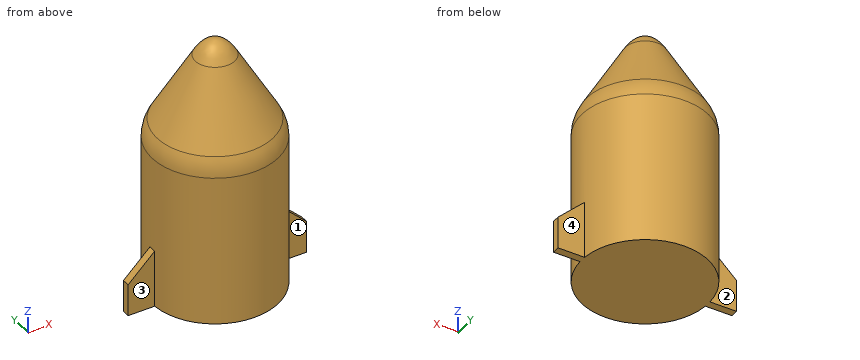
```python
from build123d import *

# Parameters (mm, degrees)
PAD_DEPTH = 1.5


with BuildPart() as part:
    # Sketch → Revolution (revolve)
    with BuildSketch(Plane.XZ):
        with BuildLine():
            Line((0, 0), (0, 100))
            add(Edge.make_bspline(
                [(7.831253, 93.75638), (4.226497, 100), (0, 100)],
                knots=[2.592301, 2.592301, 2.592301, 3.141593, 3.141593, 3.141593], degree=2, weights=[1, 0.962521, 1]))
            Line((7.831253, 93.75638), (22.990381, 67.5))
            ThreePointArc((22.990381, 67.5), (24.488887, 63.882286), (25, 60))
            Line((25, 60), (25, 0))
            Line((25, 0), (0, 0))
        make_face()
    revolve(axis=Axis((0, 0, 0), (0, 0, 1)))

    # Sketch001 → Pad (new body, symmetric)
    with BuildSketch(Plane(origin=(24, 0, 0), x_dir=(1, 0, 0), z_dir=(0, -1, 0))):
        Polygon((0, 23.592846), (11.547151, 12.692001), (11.547151, 0), (0, 0), align=None)
    pad = extrude(amount=PAD_DEPTH, both=True)

    # Mirrored: Pad across YZ
    add(pad.mirror(Plane.YZ))


solid = part.part
```
Could you check a few things on this model? Use its own coordinates, in mm. Face numbers are marked on the shaded views. A direction names the side the tool comes from. Round coordinates to 2 decimals unless told otherwise and drop trailing zeros. Write each loop counter-clockwise with the first axis right and the second up, starting at its lowest first coordinate (ties: lowest second). Pieces come first, ordered by that corner, then holes.
(1) Suppose I cut it at A-A on z = 42.5. Write out the boundary of the cut face in (x, y), and give its area (3 significant figures).
Findings below:
outline: circle Ø50 at (0, 0)
area: 1,960 mm2
(2) For pin 1 (1.5 mm diameter, centred on x = 21, y = -17.5, fed in from +Z); pin 2 (1.5 mm diameter, centred on x = -14, z = 31, fed in from -Y); pin 3 (12 mm diameter, centred on y = -11.5, z = 83.5, fed in from +X); pin 4 (10 mm diameter, centred on y = -6.5, z = 45.5, fed in from -X), each with a flat end and sliding along its axis, tell me the tip position at first contact or that it passes through.
Findings below:
pin 1: passes through
pin 2: stops at y = -21.2
pin 3: stops at x = 14.52
pin 4: stops at x = -24.95
(3) Which directions (+Z, -Z, +X, -X, +Y, -Y) give clear straight access to the entire face, cutting with the end or side of a thin tool? Please do the marked faces 1, 2, 3 and 4.
Findings below:
face 1: +Z, -Z, +X, -Y
face 2: +Z, -Z, -X, +Y
face 3: +Z, -Z, -X, -Y
face 4: +Z, -Z, +X, +Y
(4) If I drill on probe 1 along Y at (x, z) = (1, 30.5); probe 2 along X at (y, z) = (3, 65.5); probe 3 along Z at (x, y) = (-6, -3.5), over which ranges is the centre line in solid material (lowest first)?
Findings below:
probe 1: y = -24.98 to 24.98
probe 2: x = -23.77 to 23.77
probe 3: z = 0 to 95.17
(5) Suppose I cut it at B-B on z = 82. Write out the boundary of the cut face in (x, y), and give its area (3 significant figures).
Findings below:
outline: circle Ø29.24 at (0, 0)
area: 671 mm2
